Autodesk Inventor part; units mm, degrees
ref_plane "YZ Plane" through (0, 0, 0) normal (1, 0, 0) x (0, 1, 0)
ref_plane "XZ Plane" through (0, 0, 0) normal (0, 1, 0) x (-1, 0, 0)
ref_plane "XY Plane" through (0, 0, 0) normal (0, 0, 1) x (1, 0, 0)
sketch "Sketch1" plane through (0, 0, 0) normal (0, 1, 0) x (-1, 0, 0)
  circle A0 centre (0, 0) radius 6
  circle A1 centre (0, 0) radius 9.5
  circle A2 centre (6, 0) radius 1.25
  line L0 (6, 0) -> (4.0311, 0)
  circle A3 centre (4.2426, 4.2426) radius 1.25
  circle A4 centre (0, 6) radius 1.25
  circle A5 centre (-4.2426, 4.2426) radius 1.25
  circle A6 centre (-6, 0) radius 1.25
  circle A7 centre (-4.2426, -4.2426) radius 1.25
  circle A8 centre (0, -6) radius 1.25
  circle A9 centre (4.2426, -4.2426) radius 1.25
  point P0 (5.8698, -1.2432)
  point P1 (5.8698, 1.2432)
  point P2 (5.0296, -3.2715)
  point P3 (3.2715, -5.0296)
  point P4 (1.2432, -5.8698)
  point P5 (-1.2432, -5.8698)
  point P6 (-3.2715, -5.0296)
  point P7 (-5.0296, -3.2715)
  point P8 (-5.8698, -1.2432)
  point P9 (-5.8698, 1.2432)
  point P10 (-5.0296, 3.2715)
  point P11 (-3.2715, 5.0296)
  point P12 (-1.2432, 5.8698)
  point P13 (1.2432, 5.8698)
  point P14 (3.2715, 5.0296)
  point P15 (5.0296, 3.2715)
  dimension "d1" = 12
  dimension "d0" = 19
  dimension "d2" = 2.5
  dimension "d14" = 6
  dimension "d15" = 2.25
  dimension "d18" = 360
  dimension "d20" = 4.2426
  dimension "d21" = 4.2426
  dimension "d22" = 6
extrude "Extrusion1" add sketch "Sketch1" along normal blind 30
properties part number "Bearing"
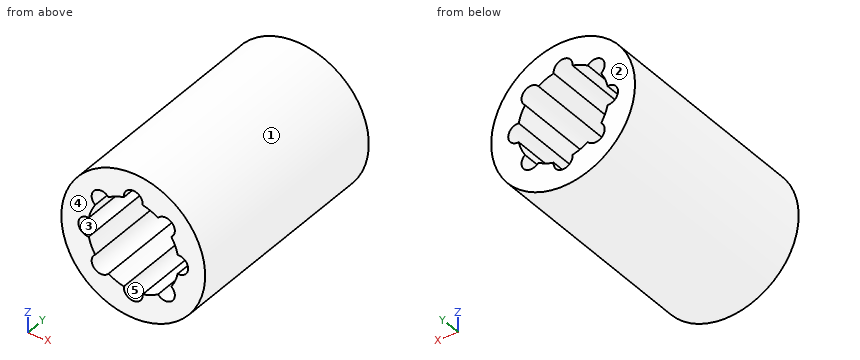
Input: part model. Units: mm. Frame: model coordinates. Face numbers are marked on the shaded views. A direction names the side the tool comes from. Give positions to 0.01 mm unless a question says otherwise; leave off trailing zeros. Loops run counter-clockwise (first coordinate to the right, second up) from the corner with the lowest first, then second, coordinate; pieces in that order, holes last. Notation, with made-up numbers: M 47.25,-14.75 L 51.25,-14.75 A20 ccw 51.25,7.25 Z; hole C 39,-34.5 d11. An arc over 180 degrees is marked long. Use one line per item in the form item = value.
1. Section query C-C, the plane y = 21. Return the cut outline in (x, z), and give its area (3 significant figures).
Numbers:
outline = C 0,0 d19; hole M -5.87,-1.24 A6 ccw -5.03,-3.27 A1.25 ccw long -3.27,-5.03 A6 ccw -1.24,-5.87 A1.25 ccw long 1.24,-5.87 A6 ccw 3.27,-5.03 A1.25 ccw long 5.03,-3.27 A6 ccw 5.87,-1.24 A1.25 ccw long 5.87,1.24 A6 ccw 5.03,3.27 A1.25 ccw long 3.27,5.03 A6 ccw 1.24,5.87 A1.25 ccw long -1.24,5.87 A6 ccw -3.27,5.03 A1.25 ccw long -5.03,3.27 A6 ccw -5.87,1.24 A1.25 ccw long Z
area = 150 mm²
2. Pull-direction query (Z, two-part tool) for the marked faces 1, 2 and 3; classes: released by +Z, released by -Z, zero draft, split by the parting line, or undercut.
Numbers:
face_1 = split by the parting line
face_2 = zero draft
face_3 = undercut
3. Section query B-B, the plane z = 6.5. Return the cut outline in (x, y), and give its area (3 significant figures).
Numbers:
outline = M -6.93,0 L -1.15,0 L -1.15,30 L -6.93,30 Z; M 1.15,0 L 6.93,0 L 6.93,30 L 1.15,30 Z
area = 347 mm²
4. Reachability of the marked faces 4 and 5 from +Z, -Z, +X, -X, +Y, -Y: full face, straight path, thin tool, end or side. Return the list, or none.
Numbers:
face_4 = +Z, -Z, +X, -X, -Y
face_5 = +Y, -Y
5. Section query A-A, the plane x = 0. Return the cut outline in (y, z), and give its area (3 significant figures).
Numbers:
outline = M 0,-9.5 L 30,-9.5 L 30,-7.25 L 0,-7.25 Z; M 0,7.25 L 30,7.25 L 30,9.5 L 0,9.5 Z
area = 135 mm²
6. Line query: L1, parallel to X at y = 9, z = -5.25; L2, parallel to Z at x = 0, y = 20.75; L3, parallel to Z at x = 4.25, y = 27. Output: solid intervals per line, ascending.
Numbers:
L1 = -7.92 to -4.98, -3.5 to -2.9, 2.9 to 3.5, 4.98 to 7.92
L2 = -9.5 to -7.25, 7.25 to 9.5
L3 = -8.5 to -5.49, 5.49 to 8.5
7. First-contact query: pin 1 (1.5 mm diameter, centred on x = 6, y = 7, fed in from -Z); pin 2 (1 mm diameter, centred on x = 6, y = 19, fed in from +Z); pin 3 (8 mm diameter, centred on y = 16, z = 4.5, fed in from +X). Flat tips, straight axial feed; report the tip coordinate or a pass-through.
Numbers:
pin_1 = -7.92
pin_2 = 7.75
pin_3 = 9.49
